For this review, take the finished solid that the model builds, in its own axes (mm). Give positions to 0.01 mm unless a question says otherwise; leave off trailing zeros. Loops run counter-clockwise (first coordinate to the right, second up) from the corner with the lowest first, then second, coordinate; pieces in that order, holes last. Notation, with made-up numbers: (-18.75, 61.5) - (3.25, 61.5) arc R14 cw to (3.25, 70.5) - close; hole circle Ø10 at (67, 2.25). An arc over 180 degrees is marked (long way). Use CSV: the item, a comma, the result in double quotes. Start each with the question number.
1. Take a section at A-A on x = 0. Give the boundary of the cut face in (y, z).
2. Take a section at C-C on y = 0. Give the boundary of the cut face in (x, z).
3. Mouldability with a two-part tool opening along Y and no side actions: class faces 1 (the flat face through (0, 7, 0)), 2 (the cylindrical face through (-5.595, -0.246, 0.986)), 3 (the flat face through (0, -7.5, 1)) as pulls with the +Y half, pulls with the -Y half, needs draft (parallel to the pull), parting line crosses it, or undercut.
4. For pin 1 (9 mm diameter, centred on x = 0, y = 0, fed in from +Z), flat-tipped, find the tip position at first contact; note if it passes through.
5. Take a section at B-B on z = 0.95. Give the boundary of the cut face in (x, y), plus the area to 3 significant figures.
6. Wall thickness on line 1 (Y direction, x = 0, z = 1.5); line 2 (X direction, y = 0, z = 0.55); line 3 (Y direction, x = -7.75, z = 0.45): over which ranges is each line inside the solid? List them lowest first.
Autodesk Inventor part; units mm, degrees
ref_plane "YZ Plane" through (0, 0, 0) normal (1, 0, 0) x (0, 1, 0)
ref_plane "XZ Plane" through (0, 0, 0) normal (0, 1, 0) x (-1, 0, 0)
ref_plane "XY Plane" through (0, 0, 0) normal (0, 0, 1) x (1, 0, 0)
sketch "Sketch1" plane through (0, 0, 0) normal (0, 0, 1) x (1, 0, 0)
  line L0 (-9.75, -4.725) -> (-9.75, 4.725)
  line L1 (9.75, 4.725) -> (9.75, -4.725)
  circle A0 centre (0, 0) radius 5.6
  line L2 (0, 0) -> (0, 7.5)
  line L3 (0, 0) -> (0, -7.5)
  line L4 (-9.75, 7.5) -> (9.75, 7.5)
  line L5 (9.75, 7.5) -> (9.75, -7.5)
  line L6 (9.75, -7.5) -> (-9.75, -7.5)
  line L7 (-9.75, -7.5) -> (-9.75, 7.5)
  point P0 (0, 0)
  dimension "d0" = 11.2
  dimension "d5" = 7.5
  dimension "d6" = 7.5
extrude "Extrusion1" add sketch "Sketch1" along normal blind 2 contours L0 L7 L4 L2 A0 L3 L6 | L3 A0 L2 L4 L5 L1 L6
sketch "Sketch2" plane through (-9.75, 7.5, 0) normal (0, 1, 0) x (1, 0, 0)
  line L0 (0, 0) -> (19.5, 0)
  line L1 (0, 0) -> (0, -2)
  line L2 (19.5, -2) -> (0, -2)
  line L3 (19.5, 0) -> (19.5, -2)
  point P0 (9.75, 0)
extrude "Extrusion2" add sketch "Sketch2" along normal blind 5
fillet "Fillet3" radius 0.5 4 edges at (-9.75, 12.5, 1) (9.75, 12.5, 1) (-9.75, -7.5, 1) (9.75, -7.5, 1)
fillet "Fillet4" radius 0.5 12 edges at (0, 12.5, 0) (9.75, 2.5, 0) (9.6036, -7.3536, 0) (0, -7.5, 0) (-9.6036, -7.3536, 0) (-9.75, 2.5, 0) (0, 12.5, 2) (9.75, 2.5, 2) (9.6036, -7.3536, 2) (0, -7.5, 2) (-9.6036, -7.3536, 2) (-9.75, 2.5, 2)
properties part number "SyringeAttachment"
Check result:
1,outline,"(-7.5, 0.5) arc R0.5 ccw to (-7, 0) - (-5.6, 0) - (-5.6, 2) - (-7, 2) arc R0.5 ccw to (-7.5, 1.5) - close; (5.6, 0) - (12, 0) arc R0.5 ccw to (12.5, 0.5) - (12.5, 1.5) arc R0.5 ccw to (12, 2) - (5.6, 2) - close"
2,outline,"(-9.75, 0.5) arc R0.5 ccw to (-9.25, 0) - (-5.6, 0) - (-5.6, 2) - (-9.25, 2) arc R0.5 ccw to (-9.75, 1.5) - close; (5.6, 0) - (9.25, 0) arc R0.5 ccw to (9.75, 0.5) - (9.75, 1.5) arc R0.5 ccw to (9.25, 2) - (5.6, 2) - close"
3,face 1,"needs draft"
3,face 2,"undercut"
3,face 3,"pulls with the -Y half"
4,pin 1,"passes through"
5,outline,"(-9.75, -7) arc R0.5 ccw to (-9.25, -7.5) - (9.25, -7.5) arc R0.5 ccw to (9.75, -7) - (9.75, 12) arc R0.5 ccw to (9.25, 12.5) - (-9.25, 12.5) arc R0.5 ccw to (-9.75, 12) - close; hole circle Ø11.2 at (0, 0)"
5,area,"291 mm²"
6,line 1,"y = -7.5 to -5.6, 5.6 to 12.5"
6,line 2,"x = -9.75 to -5.6, 5.6 to 9.75"
6,line 3,"y = -7.5 to 12.5"
